from build123d import *

# Parameters (mm, degrees)
SKETCH013_R  = 27
PAD008_DEPTH = 10
SKETCH011_W  = 8
SKETCH011_H  = 80
SKETCH011_R  = 1.5
PAD007_DEPTH = 2.5
SKETCH010_W  = 7.5
SKETCH010_H  = 80
PAD006_DEPTH = 7.5


with BuildPart() as pad008:
    # Sketch013 → Pad008 (new body)
    with BuildSketch(Plane(origin=(0, -40, 12.5), x_dir=(1, 0, 0), z_dir=(0, 0, 1))):
        Circle(SKETCH013_R)
    extrude(amount=PAD008_DEPTH)


with BuildPart() as pad007:
    # Sketch011 → Pad007 (new body)
    with BuildSketch(Plane.XY.offset(10)):
        with Locations((-4, -40)):
            Rectangle(SKETCH011_W, SKETCH011_H)
        with Locations((-4, -45)):
            Circle(SKETCH011_R, mode=Mode.SUBTRACT)
        with Locations((-4, -65)):
            Circle(SKETCH011_R, mode=Mode.SUBTRACT)
        with Locations((-4, -55)):
            Circle(SKETCH011_R, mode=Mode.SUBTRACT)
        with Locations((-4, -75)):
            Circle(SKETCH011_R, mode=Mode.SUBTRACT)
        with Locations((-4, -35)):
            Circle(SKETCH011_R, mode=Mode.SUBTRACT)
        with Locations((-4, -25)):
            Circle(SKETCH011_R, mode=Mode.SUBTRACT)
        with Locations((-4, -15)):
            Circle(SKETCH011_R, mode=Mode.SUBTRACT)
        with Locations((-4, -5)):
            Circle(SKETCH011_R, mode=Mode.SUBTRACT)
    extrude(amount=PAD007_DEPTH)


with BuildPart() as cut002:
    # Sketch010 → Pad006 (new body)
    with BuildSketch(Plane.XY.offset(10)):
        with Locations((3.75, -40)):
            Rectangle(SKETCH010_W, SKETCH010_H)
    extrude(amount=PAD006_DEPTH)

    # Fusion003: union Pad007
    add(pad007.part)


with BuildPart() as cut002_1:
    # Fusion003 placement: moved
    add(cut002.part.moved(Location((24, 5, 0))))

    # Cut002: cut Pad008
    add(pad008.part, mode=Mode.SUBTRACT)


solid = cut002_1.part
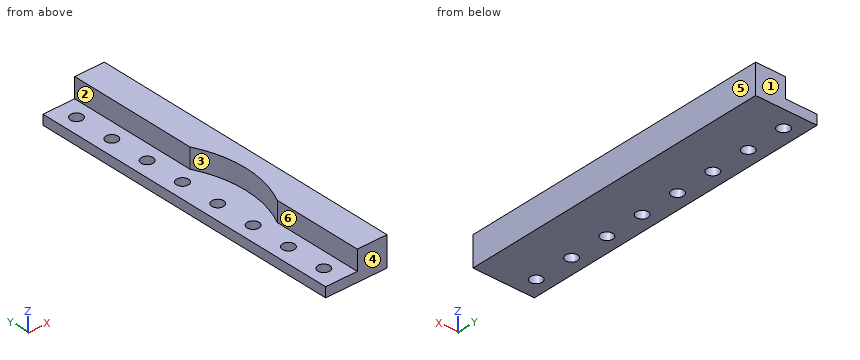
CAD build for the part. Positions are in the model's coordinates, mm. Face numbers are marked on the shaded views. A direction names the side the tool comes from. Give positions to 0.01 mm unless a question says otherwise; leave off trailing zeros. Loops run counter-clockwise (first coordinate to the right, second up) from the corner with the lowest first, then second, coordinate; pieces in that order, holes last. Notation, with made-up numbers: M 28.25,24 L 85.25,24 A33 ccw 85.25,59 Z; hole C -25.5,11.5 d2. An arc over 180 degrees is marked long. Answer in a Markdown table with one row per item. Add a question column.
Item 1: Probe probe 1 along X at (y, z) = (-60.5, 13); probe 2 along X at (y, z) = (-60, 11.15); probe 3 along Z at (x, y) = (20.5, -61.5). List the from-to ranges inside material, lowest first.
Item 2: Band-saw the part on A-A on y = -10. Give the cut face in (x, z), then the cut area to 4 significant figures.
Item 3: Band-saw the part on D-D on y = -45.5. Give the cut face in (x, z).
Item 4: Tool access for the marked faces 5 and 6: list every direction of +Z, -Z, +X, -X, +Y, -Y with a clear straight run to the whole face (end or side of a thin tool).
Item 5: Drop flat-ended pins along their axis: P1, Ø4, axis at x = 20, y = -70, coming from the +Z side; P2, Ø1.5, axis at y = -6, z = 14.5, coming from the -X side. Give the stop position or say it passes through.
Item 6: Mould opens along Y. For the marked faces 1, 2, 3 and 4 say: +Y half, -Y half, draft (parallel to the pull), parting line (faces both ways), or undercut.
Item 7: Band-saw the part on B-B on z = 11.5. Give the number of separate pieces and of enclosed holes in the cut face, then the cut area to 3 significant figures.
Reply:
| question | item | result |
|---|---|---|
| 1 | probe 1 | x = 24 to 31.5 |
| 1 | probe 2 | x = 16 to 18.5, 21.5 to 31.5 |
| 1 | probe 3 | z = 10 to 12.5 |
| 2 | outline | M 16,10 L 18.5,10 L 18.5,12.5 L 16,12.5 Z; M 21.5,10 L 31.5,10 L 31.5,17.5 L 24,17.5 L 24,12.5 L 21.5,12.5 Z |
| 2 | area | 68.75 mm^2 |
| 3 | outline | M 16,10 L 31.5,10 L 31.5,17.5 L 26.43,17.5 L 26.43,12.5 L 16,12.5 Z |
| 4 | face 5 | +Z, -Z, +X, +Y, -Y |
| 4 | face 6 | +Z, -X, +Y, -Y |
| 5 | P1 | stops at z = 12.5 |
| 5 | P2 | stops at x = 24 |
| 6 | face 1 | +Y half |
| 6 | face 2 | draft |
| 6 | face 3 | undercut |
| 6 | face 4 | -Y half |
| 7 | separate pieces | 1 |
| 7 | enclosed holes | 8 |
| 7 | area | 1,180 mm^2 |
